Autodesk Inventor part; units mm, degrees
ref_plane "YZ Plane" through (0, 0, 0) normal (1, 0, 0) x (0, 1, 0)
ref_plane "XZ Plane" through (0, 0, 0) normal (0, 1, 0) x (-1, 0, 0)
ref_plane "XY Plane" through (0, 0, 0) normal (0, 0, 1) x (1, 0, 0)
sketch "Sketch1" plane through (0, 0, 0) normal (0, 0, 1) x (1, 0, 0)
  line L0 (-12.5, 20) -> (12.5, 20)
  line L1 (12.5, 20) -> (12.5, -20)
  line L2 (12.5, -20) -> (-12.5, -20)
  line L3 (-12.5, -20) -> (-12.5, 20)
  point P0 (0, 0)
  point P1 (-12.5, 0)
  point P2 (0, 20)
  dimension "d0" = 40
  dimension "d1" = 25
extrude "Extrusion1" add sketch "Sketch1" along normal blind 15
sketch "Sketch3" plane through (0, 0, 15) normal (0, 0, -1) x (-1, 0, 0)
  line L0 (-12.5, -20) -> (-12.5, 20)
  line L1 (-12.5, -20) -> (-12.5, 20)
  line L2 (12.5, -20) -> (-12.5, -20)
  line L3 (-12.5, 20) -> (12.5, 20)
  line L4 (0, 0) -> (0, 4.9357) construction
  point P0 (-7, -14)
  point P1 (-7, 14)
  point P2 (0, -20)
  point P3 (0, 20)
  point P4 (7, -14)
  point P5 (7, 14)
  dimension "d21" = 6
  dimension "d22" = 6
  dimension "d24" = 5.5
hole "Hole1" at (7, -14, 15) at (-7, -14, 15) at (-7, 14, 15) at (7, 14, 15) direction (0, 0, -1) diameter 5 end through all counterbore diameter 10 counterbore depth 5
sketch "Sketch4" plane through (0, 0, 15) normal (0, 0, 1) x (1, 0, 0)
  line L0 (-12.5, 5) -> (12.5, 5)
  line L1 (12.5, 5) -> (12.5, -5)
  line L2 (12.5, -5) -> (-12.5, -5)
  line L3 (-12.5, -5) -> (-12.5, 5)
  line L4 (12.5, -20) -> (12.5, 20)
  line L5 (-12.5, 20) -> (-12.5, -20)
  point P0 (0, 0)
  point P1 (12.5, 0)
  dimension "d20" = 10
extrude "Extrusion3" add sketch "Sketch4" along normal blind 25
sketch "Sketch5" plane through (-12.5, 5, 15) normal (0, 1, 0) x (1, 0, 0)
  circle A0 centre (10, -13) radius 6
  line L0 (25, -25) -> (0, -25)
  line L1 (25, 0) -> (25, -25)
  circle A1 centre (10, -5) radius 1.75
  circle A2 centre (2, -13) radius 1.75
  circle A3 centre (10, -21) radius 1.75
  circle A4 centre (18, -13) radius 1.75
  point P0 (12.5, 15)
  dimension "d27" = 12
  dimension "d28" = 12
  dimension "d29" = 15
  dimension "d30" = 3.5
  dimension "d31" = 8
  dimension "d34" = 360
extrude "Extrusion4" cut sketch "Sketch5" against normal through all
fillet "Fillet2" radius 2 2 edges at (0, 5, 15) (0, -5, 15)
sketch "Sketch6" plane through (0, 0, 15) normal (0, 0, 1) x (1, 0, 0)
  line L0 (12.5, 7) -> (12.5, 20)
  line L1 (12.5, 9) -> (7, 9)
  circle A0 centre (7, 14) radius 5
  line L2 (2, 14) -> (2, 20)
  line L3 (12.5, 20) -> (-12.5, 20)
  point P0 (0, 0)
extrude "Extrusion5" cut sketch "Sketch6" against normal up to surface (5 mm away) contours L1 A0 L2 L3 L0
mirror "Mirror1" about plane through (0, 0, 0) normal (1, 0, 0) of "Extrusion5"
mirror "Mirror2" about plane through (0, 0, 0) normal (0, 1, 0) of "Extrusion5", "Mirror1"
sketch "Sketch7" plane through (-12.5, 5, 40) normal (0, 1, 0) x (1, 0, 0)
  circle A0 centre (10, 4) radius 1.75
  circle A1 centre (18, 12) radius 1.75
  circle A2 centre (10, 20) radius 1.75
  circle A3 centre (2, 12) radius 1.75
  circle A4 centre (10, 12) radius 6
  line L0 (0, 23) -> (0, 0)
  line L1 (11, 5.4361) -> (11, 6.0839)
  line L2 (9, 5.4361) -> (9, 6.0839)
  line L3 (25, 23) -> (25, 0)
  point P0 (12.5, 40)
  dimension "d41" = 1
  dimension "d42" = 1
extrude "Extrusion6" cut sketch "Sketch7" against normal through all contours A0 L2 A4 L1
pattern_circular "Circular Pattern1" count 4 over 360 about axis through (-2.5, 5, 28) along (0, -1, 0) of "Extrusion6"
equation "\"d42\" = d41"
properties part number "0008-10-013 Supăort Piulita Axa Z1"
Design review of the part built by this model. Coordinates are the model's own, in mm. A direction names the side the tool comes from. Round coordinates to 2 decimals unless told otherwise and drop trailing zeros. Write each loop counter-clockwise with the first axis right and the second up, starting at its lowest first coordinate (ties: lowest second). Pieces come first, ordered by that corner, then holes.
Item 1: Draft analysis for pull direction Z (two halves, no side actions). For faces 4 (the flat face through (-10, -15, 10)), 5 (the cylindrical face through (1.779, 0.07, 23.794)), 6 (the flat face through (-2, -17, 13)), state which applies: released by +Z, released by -Z, zero draft, split by the parting line, or undercut.
Item 2: Consider section C-C on x = 10.25. Give the boundary of the cut face in (y, z), and give its area (3 significant figures).
Item 3: Wall thickness on L1, parallel to X at y = -14, z = 5; L2, parallel to Y at x = -7, z = 4.5; L3, parallel to Z at x = 5.5, y = -0.75: over which ranges is each line inside the solid? List them lowest first.
Item 4: Consider section B-B on y = 16. Give the boundary of the cut face in (x, z), and give its area (3 significant figures).
Item 5: Consider section A-A on z = 36. Give the boundary of the cut face in (x, y), and give its area (3 significant figures).
Item 6: Consider section D-D on y = 4.5. Give the boundary of the cut face in (x, z), and give its area (3 significant figures).
Item 7: For faces 1 (the cylindrical face through (-4, -10, 12)), 2 (the cylindrical face through (-3, 11, 12)), 3 (the flat face through (2, -17, 13)), list the 3-axis set-ups (+Z, -Z, +X, -X, +Y, -Y) from which the entire face can be reached by the end or side of a thin tool; tool diameter is ignored.
Item 8: For pin 1 Ø6.5 at (x, y) = (-2, 14) entering from +Z; pin 2 Ø10 at (x, z) = (-7.5, 27.5) entering from -Y; pin 3 Ø3 at (x, z) = (-2.5, 36) entering from -Y; pin 4 Ø4.5 at (x, z) = (-10.5, 28) entering from +Y, all flat-tipped, find the tip position at first contact; note any pin that passes through.
Check values:
1. face 4: released by +Z
1. face 5: undercut
1. face 6: zero draft
2. outline: (-20, 0) - (20, 0) - (20, 10) - (9, 10) - (9, 15) - (7, 15) arc R2 cw to (5, 17) - (5, 40) - (-5, 40) - (-5, 17) arc R2 cw to (-7, 15) - (-9, 15) - (-9, 10) - (-20, 10) - close
2. area: 742 mm2
3. L1: x = -12.5 to -9.5, -4.5 to 4.5, 9.5 to 12.5
3. L2: y = -20 to -16.5, -11.5 to 11.5, 16.5 to 20
3. L3: z = 0 to 26.25, 29.75 to 40
4. outline: (-12.5, 0) - (-8.5, 0) - (-8.5, 10) - (-12.5, 10) - close; (-5.5, 0) - (5.5, 0) - (5.5, 10) - (2, 10) - (2, 15) - (-2, 15) - (-2, 10) - (-5.5, 10) - close; (8.5, 0) - (12.5, 0) - (12.5, 10) - (8.5, 10) - close
4. area: 210 mm2
5. outline: (-12.5, -5) - (-4.25, -5) - (-4.25, 5) - (-12.5, 5) - close; (-0.75, -5) - (12.5, -5) - (12.5, 5) - (-0.75, 5) - close
5. area: 215 mm2
6. outline: (-12.5, 0) - (12.5, 0) - (12.5, 40) - (-12.5, 40) - close; hole (-9.06, 27) - (-8.42, 27) arc R6 ccw to (-3.5, 22.08) - (-3.5, 21.44) arc R1.75 ccw (long way) to (-1.5, 21.44) - (-1.5, 22.08) arc R6 ccw to (3.42, 27) - (4.06, 27) arc R1.75 ccw (long way) to (4.06, 29) - (3.42, 29) arc R6 ccw to (-1.5, 33.92) - (-1.5, 34.56) arc R1.75 ccw (long way) to (-3.5, 34.56) - (-3.5, 33.92) arc R6 ccw to (-8.42, 29) - (-9.06, 29) arc R1.75 ccw (long way) to start
6. area: 845 mm2
7. face 1: +Z, -X, -Y
7. face 2: +Z, -X, +Y
7. face 3: +Z, +X, -Y
8. pin 1: stops at z = 15
8. pin 2: stops at y = -5
8. pin 3: passes through
8. pin 4: stops at y = 5
